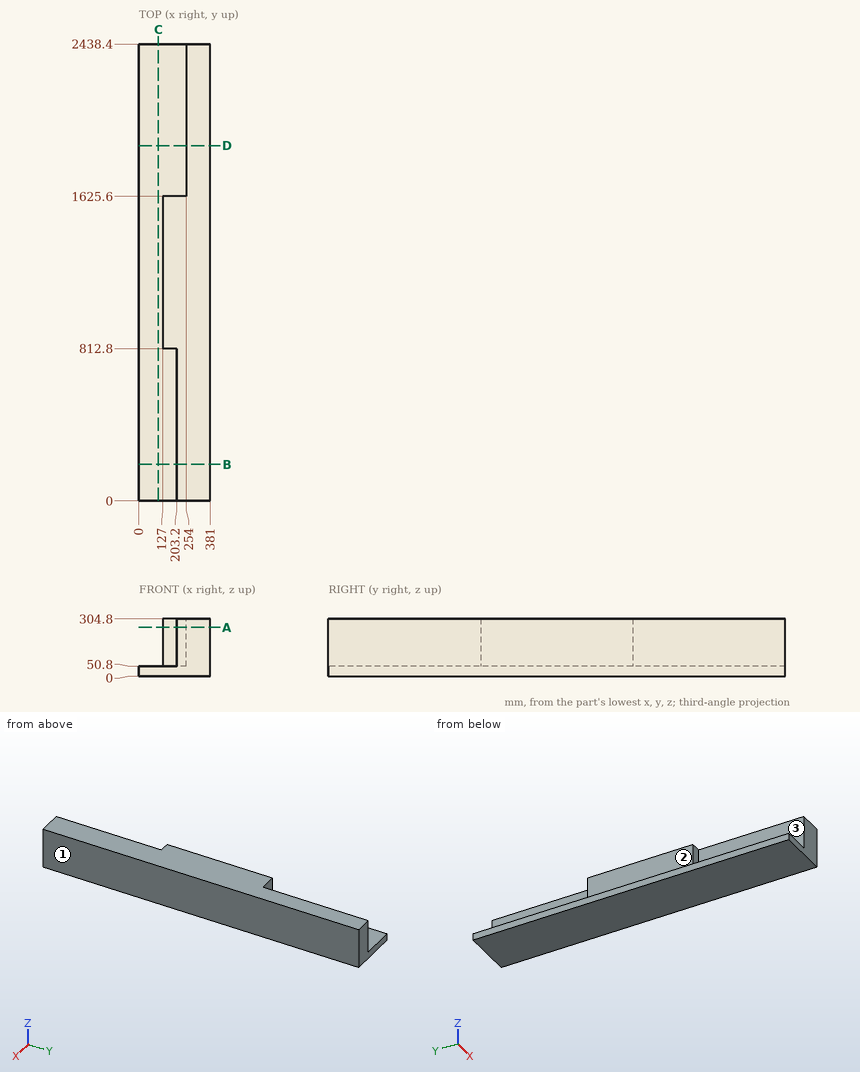
Study the drawing (mm; zero at the part's minimum x, y, z) and answer. A direction names the side the tool comes from. Coordinates: 2 decimals unless noted, no trailing zeros. Write each loop counter-clockwise with the first axis right and the second up, starting at its lowest first coordinate (ties: lowest second). Pieces come first, ordered by that corner, then holes. Notation, with made-up numbers: (36.5, 28) - (46.5, 28) arc R20 cw to (46.5, 56) - close; hole circle Ø9 at (-32.75, 45.25). An arc over 180 degrees is marked (long way). One line per item, written item: value.
1) Find section D-D (y = 1896). Give the vertices of the cut face in (x, z), and give its area (3 significant figures).
Geometry check:
outline: (0, 0) - (381, 0) - (381, 304.8) - (254, 304.8) - (254, 50.8) - (0, 50.8) - close
area: 51,600 mm2
2) A tool of negligible diameter and unlimited length cuts with its end or side. For the marked faces 1, 2 and 3, from which of +Z, -Z, +X, -X, +Y, -Y can it reach the whole face along a straight path? Write none if from no direction.
Geometry check:
face 1: +Z, -Z, +X, +Y, -Y
face 2: +Z, -X, +Y, -Y
face 3: +Z, -X, -Y
3) Find section B-B (y = 195). Give the vertices of the cut face in (x, z).
Geometry check:
outline: (0, 0) - (381, 0) - (381, 304.8) - (203.2, 304.8) - (203.2, 50.8) - (0, 50.8) - close
4) Each of these flat-tipped pins is pushed along its axis until it touches: pin 1 Ø4 at (x, z) = (284, 91.5) entering from -Y; pin 2 Ø10 at (y, z) = (292, 143) entering from -X; pin 3 Ø12 at (y, z) = (1533.5, 125) entering from -X. Where does it stop, or does it pass through?
Geometry check:
pin 1: stops at y = 0
pin 2: stops at x = 203.2
pin 3: stops at x = 127
5) Find section C-C (x = 104.5). Give the vertices of the cut face in (y, z), and give its area (3 significant figures).
Geometry check:
outline: (0, 0) - (2438.4, 0) - (2438.4, 50.8) - (0, 50.8) - close
area: 124,000 mm2
6) Consider line 1 along X through (y, z) = (2282, 217.5); line 2 along X through (y, z) = (554.5, 269.5); line 3 along Y through (x, z) = (241.5, 94.5). Determine where each line is inside the solid, lowest interval first. Write a range as from..to.
Geometry check:
line 1: x = 254..381
line 2: x = 203.2..381
line 3: y = 0..1625.6
7) Find section A-A (z = 259). Give the vertices of the cut face in (x, y), and give its area (3 significant figures).
Geometry check:
outline: (127, 812.8) - (203.2, 812.8) - (203.2, 0) - (381, 0) - (381, 2438.4) - (254, 2438.4) - (254, 1625.6) - (127, 1625.6) - close
area: 454,000 mm2
